Could you check a few things on this drawing? It's one solid part, dimensions in mm from its lowest x, y, z. Round coordinates to 2 decimals unless told otherwise and drop trailing zeros. Write each loop counter-clockwise with the first axis right and the second up, starting at its lowest first coordinate (ties: lowest second). Pieces come first, ordered by that corner, then holes. Notation, with made-up numbers: (10, -0.75) -> (60, -0.75) arc R19 cw to (60, 10.25) -> close; hole circle Ø4 at (-21, 46.5). An arc over 180 degrees is marked (long way). Answer in a Markdown table with one row per item.
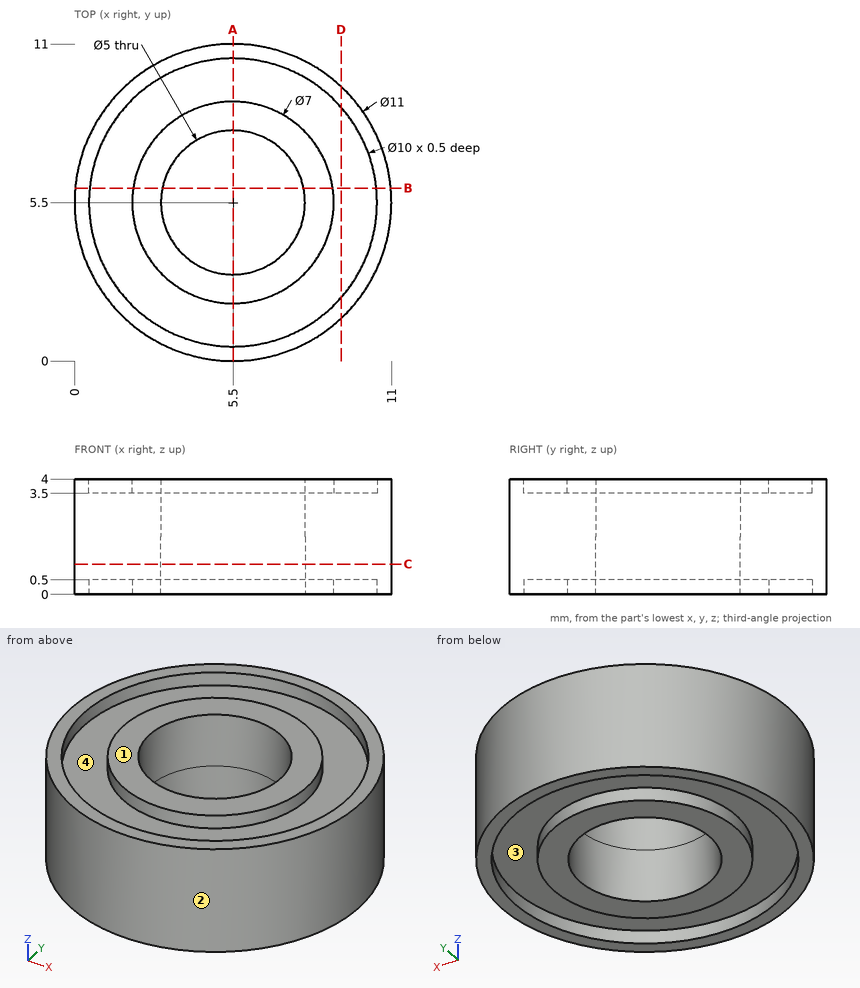
1) Imagine slicing it at A-A, the plane x = 5.5. Please give me the cut outline in (y, z), plus the area to 3 significant figures.
Findings:
| item | result |
|---|---|
| outline | (0, 0) -> (0.5, 0) -> (0.5, 0.5) -> (2, 0.5) -> (2, 0) -> (3, 0) -> (3, 4) -> (2, 4) -> (2, 3.5) -> (0.5, 3.5) -> (0.5, 4) -> (0, 4) -> close; (8, 0) -> (9, 0) -> (9, 0.5) -> (10.5, 0.5) -> (10.5, 0) -> (11, 0) -> (11, 4) -> (10.5, 4) -> (10.5, 3.5) -> (9, 3.5) -> (9, 4) -> (8, 4) -> close |
| area | 21.0 mm^2 |
2) For pin 1 (3 mm diameter, centred on x = 1.5, y = 4, fed in from +Z); pin 2 (1 mm diameter, centred on x = 6.5, y = 4.5, fed in from +Z); pin 3 (1.5 mm diameter, centred on y = 9.5, z = 2.5, fed in from -X); pin 4 (1 mm diameter, centred on x = 8.5, z = 2.5, fed in from +Y), each with a flat end and sliding along its axis, tell me the tip position at first contact or that it passes through.
Findings:
| item | result |
|---|---|
| pin 1 | stops at z = 4 |
| pin 2 | passes through |
| pin 3 | stops at x = 1.06 |
| pin 4 | stops at y = 10.4 |
3) Please list where these lines run through material, in increasing order: line 1 (X direction, y = 8.5, z = 0.4); line 2 (Z direction, x = 8.5, y = 2.25); line 3 (Y direction, x = 5.5, z = 2.7).
Findings:
| item | result |
|---|---|
| line 1 | x = 0.89 to 1.5, 3.7 to 7.3, 9.5 to 10.11 |
| line 2 | z = 0.5 to 3.5 |
| line 3 | y = 0 to 3, 8 to 11 |
4) Thinking about a two-plate mould opening in Y: for the marked faces 1, 2, 3 and 4, which applies, +Y half, -Y half, draft (parallel to the pull), parting line (faces both ways), or undercut?
Findings:
| item | result |
|---|---|
| face 1 | draft |
| face 2 | parting line |
| face 3 | undercut |
| face 4 | undercut |
5) Imagine slicing it at D-D, the plane x = 9.25. Please give me the cut outline in (y, z), plus the area to 3 significant figures.
Findings:
| item | result |
|---|---|
| outline | (1.48, 0) -> (2.19, 0) -> (2.19, 0.5) -> (8.81, 0.5) -> (8.81, 0) -> (9.52, 0) -> (9.52, 4) -> (8.81, 4) -> (8.81, 3.5) -> (2.19, 3.5) -> (2.19, 4) -> (1.48, 4) -> close |
| area | 25.6 mm^2 |
6) Imagine slicing it at C-C, the plane z = 1.05. Please give me the cut outline in (x, y).
Findings:
| item | result |
|---|---|
| outline | circle Ø11 at (5.5, 5.5); hole circle Ø5 at (5.5, 5.5) |
7) Imagine slicing it at B-B, the plane y = 6. Please give me the cut outline in (x, z), plus the area to 3 significant figures.
Findings:
| item | result |
|---|---|
| outline | (0.02, 0) -> (0.53, 0) -> (0.53, 0.5) -> (2.04, 0.5) -> (2.04, 0) -> (3.05, 0) -> (3.05, 4) -> (2.04, 4) -> (2.04, 3.5) -> (0.53, 3.5) -> (0.53, 4) -> (0.02, 4) -> close; (7.95, 0) -> (8.96, 0) -> (8.96, 0.5) -> (10.47, 0.5) -> (10.47, 0) -> (10.98, 0) -> (10.98, 4) -> (10.47, 4) -> (10.47, 3.5) -> (8.96, 3.5) -> (8.96, 4) -> (7.95, 4) -> close |
| area | 21.2 mm^2 |
